The listing builds one solid part. Answer for the finished solid, in the listing's coordinates (mm). A direction names the side the tool comes from. Round coordinates to 2 decimals unless told otherwise and drop trailing zeros. Order: outer loops, then holes, each group sorted by start corner. A loop starts at its lowest first (then second) coordinate and runs counter-clockwise, first axis right, second up. Notation, with made-up numbers: (-19, 85) -> (19, 85) arc R29 ccw to (19, 122) -> close; hole circle Ø5 at (-7.75, 44). An arc over 180 degrees is marked (long way). Return JSON: item names as keys, results as strings. Group by question number.
(1) Determine the mould class of faces 4 (the face through (-30, 61, 9)), 5 (the face through (-3, 27, 18)), 6 (the face through (-202.708, 33.376, 8.874)) for opening direction X: +X half, -X half, draft (parallel to the pull), parting line (faces both ways), or undercut.
(2) The part is cut by section B-B (z = 14.5). Determine the outline of the cut face in (x, y), plus the area to 3 significant figures.
(3) The part is cut by section C-C (x = -105.5). Determine the outline of the cut face in (y, z), plus the area to 3 significant figures.
(4) Which of the six approach directions +Z, -Z, +X, -X, +Y, -Y give full straight-line access (tool end or side, diameter ignored) to faces 1 (the face through (-84, 55, 9)), 2 (the face through (-195.62, 4.47, 8.87)), 3 (the face through (-3, 27, 0))?
(5) Consider line 1 (Y direction, x = -114, z = 6.5); line 2 (X direction, y = 11, z = 8.25); line 3 (X direction, y = 30, z = 16). Determine where each line is inside the solid, lowest interval first. Write a range as [from, to].
(6) The part is cut by section A-A (y = 59). Determine the outline of the cut face in (x, z).
(7) The part is cut by section D-D (y = 35). Determine the outline of the cut face in (x, z), plus the area to 3 significant figures.
(8) Each of these flat-tipped pins is pushed along its axis until it touches: pin 1 (6 mm diameter, centred on y = 58.5, z = 11, fed in from +X); pin 2 (1.5 mm diameter, centred on y = 30, z = 13.5, fed in from -X); pin 3 (9 mm diameter, centred on x = -104.5, z = 11.5, fed in from +Y). Where does it stop, or does it pass through?
from build123d import *

# Parameters (mm, degrees)
PAD_DEPTH = 18


with BuildPart() as part:
    # Sketch → Pad (new body)
    with BuildSketch(Plane.XY):
        Polygon((0, 67), (30, 67), (30, 55), (140, 55), (185.301157, 62.987816), (187.037638, 53.139739), (198.855331, 55.223517), (206.669499, 10.907168), (194.851806, 8.82339), (196.407608, 0), (0, 0), align=None)
    pad = extrude(amount=PAD_DEPTH)

    # Mirrored: Pad across Sketch V_Axis
    add(pad.mirror(Plane(origin=(0, 0, 0), x_dir=(0, 0, 1), z_dir=(1, 0, 0))))


solid = part.part
Answer below:
{
 "1": {"face 4": "undercut", "face 5": "draft", "face 6": "-X half"},
 "2": {"outline": "(-206.67, 10.91) -> (-194.85, 8.82) -> (-196.41, 0) -> (196.41, 0) -> (194.85, 8.82) -> (206.67, 10.91) -> (198.86, 55.22) -> (187.04, 53.14) -> (185.3, 62.99) -> (140, 55) -> (30, 55) -> (30, 67) -> (-30, 67) -> (-30, 55) -> (-140, 55) -> (-185.3, 62.99) -> (-187.04, 53.14) -> (-198.86, 55.22) -> close", "area": "23,200 mm²"},
 "3": {"outline": "(0, 0) -> (55, 0) -> (55, 18) -> (0, 18) -> close", "area": "990 mm²"},
 "4": {"face 1": "+Z, -Z, +Y", "face 2": "+Z, -Z, -X", "face 3": "-Z, +X, -X, +Y, -Y"},
 "5": {"line 1": "y = [0, 55]", "line 2": "x = [-206.65, 206.65]", "line 3": "x = [-203.3, 203.3]"},
 "6": {"outline": "(-186, 0) -> (-162.69, 0) -> (-162.69, 18) -> (-186, 18) -> close; (-30, 0) -> (30, 0) -> (30, 18) -> (-30, 18) -> close; (162.69, 0) -> (186, 0) -> (186, 18) -> (162.69, 18) -> close"},
 "7": {"outline": "(-202.42, 0) -> (202.42, 0) -> (202.42, 18) -> (-202.42, 18) -> close", "area": "7,290 mm²"},
 "8": {"pin 1": "stops at x = 186.62", "pin 2": "stops at x = -203.44", "pin 3": "stops at y = 55"}
}
